Read the model definition and answer for the solid it produces. Units are mm, in the model's axes. Round coordinates to 2 decimals unless told otherwise and drop trailing zeros. Write each loop counter-clockwise with the first axis right and the second up, starting at its lowest first coordinate (ties: lowest second). Pieces come first, ordered by that corner, then holes. Notation, with made-up numbers: (71.25, 42) - (105.25, 42) arc R30 cw to (105.25, 66) - close; hole circle Ø3 at (65, -35). An arc over 180 degrees is marked (long way). Use one line per item in the form item = value. Start each with the question number.
1) The part is cut by section C-C, the plane y = -6.5. Count the separate pieces of the cut face and the enclosed holes in it, plus the area to 3 significant figures.
2) Each of these flat-tipped pins is pushed along its axis until it touches: pin 1 (1 mm diameter, centred on x = 56, y = -10, fed in from +Z); pin 2 (4 mm diameter, centred on y = -11, z = 98, fed in from +X); pin 3 (1 mm diameter, centred on y = -10, z = 148.5, fed in from +X). Where does it stop, or does it pass through?
3) Consider line 1 along Z through (x, y) = (-64, -2.5); line 2 along Z through (x, y) = (33, -0.5) (3 decimals); line 3 along X through (y, z) = (-0.75, -5.5). Determine where each line is inside the solid, lowest interval first. Write a range as from..to.
4) The part is cut by section B-B, the plane z = 68. Give the vertices of the cut face in (x, y).
5) The part is cut by section A-A, the plane x = 76.2. Give the vertices of the cut face in (y, z), plus the area to 3 significant figures.
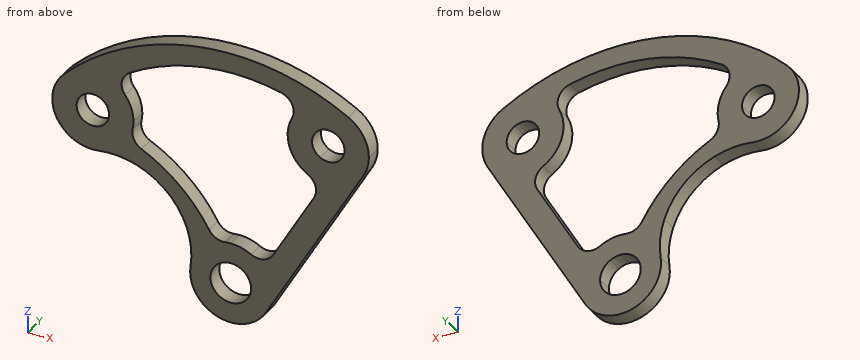
from build123d import *

# Parameters (mm, degrees)
F1_DEPTH = 12.7


with BuildPart() as f1:
    # F0 (on Front) → F1 (new body)
    with BuildSketch(Plane.XZ):
        with BuildLine():
            ThreePointArc((-76.6615778684, 102.701242205), (-79.8079393943, 94.0332154271), (-85.3124331502, 86.6349164629))
            Line((-85.3124331502, 86.6349164629), (-73.4535511858, 74.7760344986))
            ThreePointArc((-73.4535511858, 74.7760344986), (-49.3914086659, 59.6941480997), (-34.309522267, 35.6320055797))
            Line((-34.309522267, 35.6320055797), (-22.4506403027, 23.7731236154))
            ThreePointArc((-22.4506403027, 23.7731236154), (-14.0635457715, 29.7878865302), (-4.1903736131, 32.7947452108))
            ThreePointArc((-4.1903736131, 32.7947452108), (-11.4735568319, 33.9884241162), (-16.8631754222, 39.0304116786))
            ThreePointArc((-16.8631754222, 39.0304116786), (-39.690876035, 67.8137699888), (-69.8640218822, 88.7700793147))
            ThreePointArc((-69.8640218822, 88.7700793147), (-75.6347361649, 94.5783008286), (-76.6615778684, 102.701242205))
        make_face()
        with BuildLine():
            Line((-73.4535511858, 74.7760344986), (-85.3124331502, 86.6349164629))
            ThreePointArc((-85.3124331502, 86.6349164629), (-93.5640417957, 80.6874934513), (-103.2729453923, 77.6546603418))
            ThreePointArc((-103.2729453923, 77.6546603418), (-88.1910589934, 77.9990389332), (-73.4535511858, 74.7760344986))
        make_face()
        with BuildLine():
            Line((-22.4506403027, 23.7731236154), (-34.309522267, 35.6320055797))
            ThreePointArc((-34.309522267, 35.6320055797), (-31.0865178324, 20.8944977722), (-31.4308964237, 5.8126113733))
            ThreePointArc((-31.4308964237, 5.8126113733), (-28.3980633142, 15.5215149699), (-22.4506403027, 23.7731236154))
        make_face()
        with BuildLine():
            Line((27.4963065702, -14.5525166873), (103.6963065702, 117.4297548495))
            ThreePointArc((103.6963065702, 117.4297548495), (84.417504682, 102.6366098648), (60.325, 105.8084482793))
            ThreePointArc((60.325, 105.8084482793), (66.2422579939, 98.0969275241), (64.9735226281, 88.4599256513))
            Line((64.9735226281, 88.4599256513), (33.2235226281, 33.467312511))
            ThreePointArc((33.2235226281, 33.467312511), (25.5120018728, 27.5500545171), (15.875, 28.8187898829))
            ThreePointArc((15.875, 28.8187898829), (27.4963065702, 17.1974833127), (31.75, 1.3224833127))
            ThreePointArc((31.75, 1.3224833127), (30.6681449847, -6.8950213693), (27.4963065702, -14.5525166873))
        make_face()
        with BuildLine():
            ThreePointArc((92.075, 160.8010614196), (-24.0363982973, 183.8970545347), (-130.2137137555, 131.5361970682))
            ThreePointArc((-130.2137137555, 131.5361970682), (-105.7367190454, 140.7708275994), (-82.6354727067, 128.4934464175))
            ThreePointArc((-82.6354727067, 128.4934464175), (-85.0809337208, 138.5209907043), (-79.2724649931, 147.0529081346))
            ThreePointArc((-79.2724649931, 147.0529081346), (-21.7373717549, 168.3372367219), (39.542821328, 165.5004193044))
            ThreePointArc((39.542821328, 165.5004193044), (47.9856006443, 158.4820206871), (47.8023187461, 147.5045506016))
            ThreePointArc((47.8023187461, 147.5045506016), (67.0674381234, 163.7129579133), (92.075, 160.8010614196))
        make_face()
        with BuildLine():
            ThreePointArc((-116.7433295739, 118.0658128866), (-102.9029938618, 120.8188268285), (-95.0630734528, 109.0855567656))
            ThreePointArc((-95.0630734528, 109.0855567656), (-96.0298033899, 104.2254771745), (-98.7828173318, 100.1053006445))
            Line((-98.7828173318, 100.1053006445), (-85.3124331502, 86.6349164629))
            ThreePointArc((-85.3124331502, 86.6349164629), (-79.8079393943, 94.0332154271), (-76.6615778684, 102.701242205))
            ThreePointArc((-76.6615778684, 102.701242205), (-76.175615619, 105.8769733404), (-76.0130734528, 109.0855567656))
            ThreePointArc((-76.0130734528, 109.0855567656), (-77.7142479875, 119.338877601), (-82.6354727067, 128.4934464175))
            ThreePointArc((-82.6354727067, 128.4934464175), (-105.7367190454, 140.7708275994), (-130.2137137555, 131.5361970682))
            Line((-130.2137137555, 131.5361970682), (-116.7433295739, 118.0658128866))
        make_face()
        with BuildLine():
            ThreePointArc((107.95, 133.3047548495), (103.6963065702, 149.1797548495), (92.075, 160.8010614196))
            Line((92.075, 160.8010614196), (82.55, 144.3032774775))
            ThreePointArc((82.55, 144.3032774775), (87.1985226281, 139.6547548495), (88.9, 133.3047548495))
            ThreePointArc((88.9, 133.3047548495), (82.55, 122.3062322214), (69.85, 122.3062322214))
            Line((69.85, 122.3062322214), (60.325, 105.8084482793))
            ThreePointArc((60.325, 105.8084482793), (84.417504682, 102.6366098648), (103.6963065702, 117.4297548495))
            ThreePointArc((103.6963065702, 117.4297548495), (106.8681449847, 125.0872501675), (107.95, 133.3047548495))
        make_face()
        with BuildLine():
            Line((82.55, 144.3032774775), (92.075, 160.8010614196))
            ThreePointArc((92.075, 160.8010614196), (67.0674381234, 163.7129579133), (47.8023187461, 147.5045506016))
            ThreePointArc((47.8023187461, 147.5045506016), (45.7917969362, 124.1721929729), (60.325, 105.8084482793))
            Line((60.325, 105.8084482793), (69.85, 122.3062322214))
            ThreePointArc((69.85, 122.3062322214), (65.2014773719, 139.6547548495), (82.55, 144.3032774775))
        make_face()
        with BuildLine():
            ThreePointArc((-98.7828173318, 100.1053006445), (-116.7433295739, 100.1053006445), (-116.7433295739, 118.0658128866))
            Line((-116.7433295739, 118.0658128866), (-130.2137137555, 131.5361970682))
            ThreePointArc((-130.2137137555, 131.5361970682), (-136.1611367671, 94.8865251084), (-103.2729453923, 77.6546603418))
            ThreePointArc((-103.2729453923, 77.6546603418), (-93.5640417957, 80.6874934513), (-85.3124331502, 86.6349164629))
            Line((-85.3124331502, 86.6349164629), (-98.7828173318, 100.1053006445))
        make_face()
        with BuildLine():
            ThreePointArc((-4.1903736131, 32.7947452108), (-14.0635457715, 29.7878865302), (-22.4506403027, 23.7731236154))
            Line((-22.4506403027, 23.7731236154), (-11.2253201513, 12.5478034641))
            ThreePointArc((-11.2253201513, 12.5478034641), (-6.0750994888, 15.9890708914), (0, 17.1974833127))
            Line((0, 17.1974833127), (0, 33.0724833127))
            ThreePointArc((0, 33.0724833127), (-2.0997838859, 33.0029726971), (-4.1903736131, 32.7947452108))
        make_face()
        with BuildLine():
            Line((7.9375, 15.0706365978), (15.875, 28.8187898829))
            ThreePointArc((15.875, 28.8187898829), (8.217504682, 31.9906282974), (0, 33.0724833127))
            Line((0, 33.0724833127), (0, 17.1974833127))
            ThreePointArc((0, 17.1974833127), (4.108752341, 16.6565558051), (7.9375, 15.0706365978))
        make_face()
        with BuildLine():
            Line((-11.2253201513, 12.5478034641), (-22.4506403027, 23.7731236154))
            ThreePointArc((-22.4506403027, 23.7731236154), (-28.3980633142, 15.5215149699), (-31.4308964237, 5.8126113733))
            ThreePointArc((-31.4308964237, 5.8126113733), (-10.3708659021, -28.6859761686), (27.4963065702, -14.5525166873))
            ThreePointArc((27.4963065702, -14.5525166873), (30.6681449847, -6.8950213693), (31.75, 1.3224833127))
            ThreePointArc((31.75, 1.3224833127), (27.4963065702, 17.1974833127), (15.875, 28.8187898829))
            Line((15.875, 28.8187898829), (7.9375, 15.0706365978))
            ThreePointArc((7.9375, 15.0706365978), (13.7481532851, 9.2599833127), (15.875, 1.3224833127))
            ThreePointArc((15.875, 1.3224833127), (-6.0750994888, -13.3441042659), (-11.2253201513, 12.5478034641))
        make_face()
    extrude(amount=F1_DEPTH)


solid = f1.part
Geometry results:
q1.separate_pieces = 1
q1.enclosed_holes = 4
q1.area = 14,500 mm2
q2.pin_1 = 176.91
q2.pin_2 = 93.63
q2.pin_3 = 104.34
q3.line_1 = 70.6..85.67, 155.36..173.99
q3.line_2 = -5.02..33.095, 166.996..182.492
q3.line_3 = -31.01..-14.33, 14.33..32.72
q4.outline = (-59.63, -12.7) - (-39.89, -12.7) - (-39.89, 0) - (-59.63, 0) - close; (53.16, -12.7) - (75.16, -12.7) - (75.16, 0) - (53.16, 0) - close
q5.outline = (-12.7, 69.8) - (0, 69.8) - (0, 120.6) - (-12.7, 120.6) - close; (-12.7, 146) - (0, 146) - (0, 168.97) - (-12.7, 168.97) - close
q5.area = 937 mm2
